The figure shows three views and two pictorial views of one solid part (mm, origin at its lowest corner). Answer the questions. A direction names the side the tool comes from. Round coordinates to 2 decimals unless told otherwise and drop trailing zeros. Write each loop counter-clockwise with the first axis right and the second up, starting at its lowest first coordinate (ties: lowest second). Pieces come first, ordered by that corner, then holes.
Item 1: Find the intervals of material crossed by probe 1 along Z at (x, y) = (19.5, 4) (1 decimal); probe 2 along X at (y, z) = (27.5, 33.5); probe 3 along X at (y, z) = (48.5, 35.5) (1 decimal), in increasing order.
Item 2: Find section C-C on z = 36. Give the vertices of the cut face in (x, y).
Item 3: Find section A-A on x = 79. Give the vertices of the cut face in (y, z) (1 decimal).
Item 4: A tool of negligible diameter and unlimited length cuts with its end or side. For the marked faces 4, 5 and 6, from which of +Z, -Z, +X, -X, +Y, -Y can it reach the whole face along a straight path? Write none if from no direction.
Item 5: Each of these flat-tipped pins is pushed along its axis until it touches: pin 1 (6 mm diameter, centred on x = 14.5, z = 49, fed in from -Y); pin 2 (1.5 mm diameter, centred on y = 14, z = 24.5, fed in from -X). Where does it stop, or does it pass through?
Item 6: For a pull along Z with two mould halves and no side action, classify the marked faces 1, 2 and 3 as +Z half, -Z half, draft (parallel to the pull), parting line (faces both ways), or undercut.
Item 7: Find section B-B on y = 49. Give the vertices of the cut face in (x, z) (1 decimal).
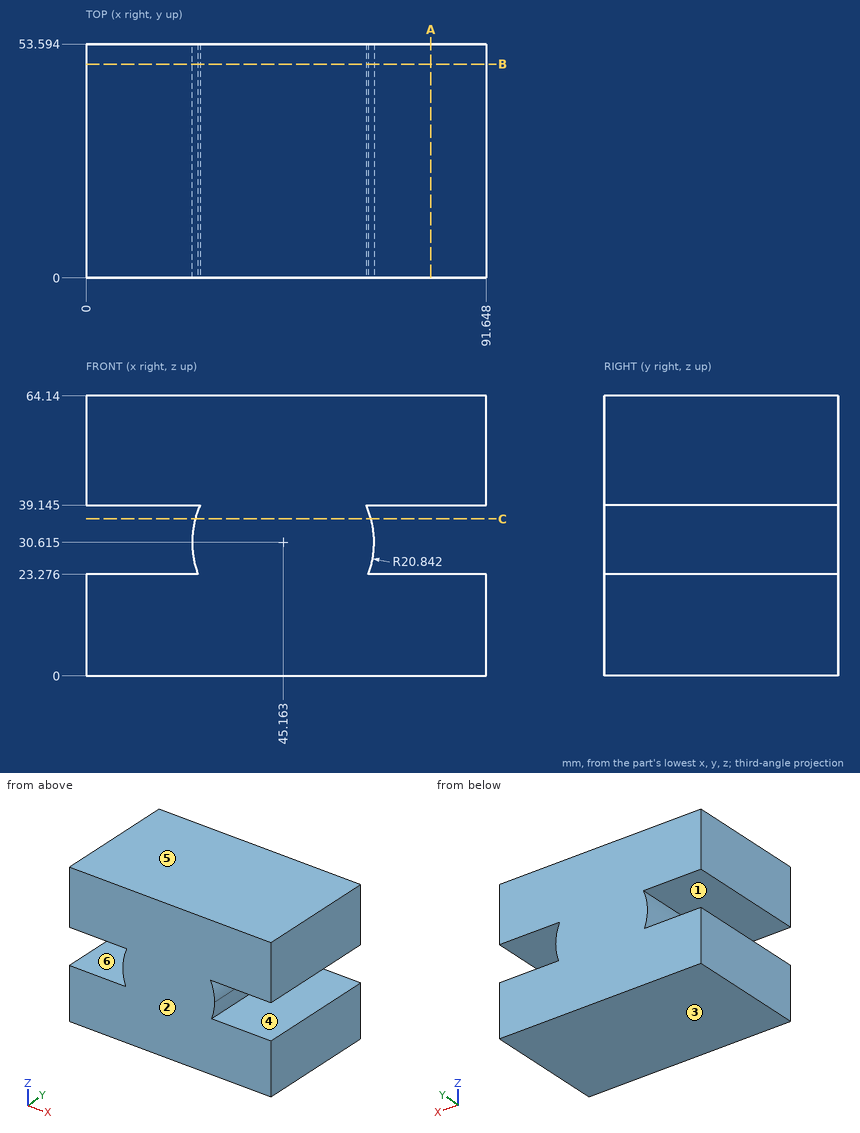
Check values:
1. probe 1: z = 0 to 23.3, 39.1 to 64.1
1. probe 2: x = 24.52 to 65.8
1. probe 3: x = 24.9 to 65.4
2. outline: (25.03, 0) - (65.3, 0) - (65.3, 53.59) - (25.03, 53.59) - close
3. outline: (0, 0) - (53.6, 0) - (53.6, 23.3) - (0, 23.3) - close; (0, 39.1) - (53.6, 39.1) - (53.6, 64.1) - (0, 64.1) - close
4. face 4: +X, +Y, -Y
4. face 5: +Z, +X, -X, +Y, -Y
4. face 6: -X, +Y, -Y
5. pin 1: stops at y = 0
5. pin 2: stops at x = 25.02
6. face 1: undercut
6. face 2: draft
6. face 3: -Z half
7. outline: (0, 0) - (91.6, 0) - (91.6, 23.3) - (64.7, 23.3) arc R20.8 ccw to (66, 30.6) arc R20.8 ccw to (64.2, 39.1) - (91.6, 39.1) - (91.6, 64.1) - (0, 64.1) - (0, 39.1) - (26.1, 39.1) arc R20.8 ccw to (25.7, 23.3) - (0, 23.3) - close
